Build history of the part. All positions in model axes, mm. Face numbers are marked on the shaded views. A direction names the side the tool comes from. Give positions to 0.01 mm unless a question says otherwise; leave off trailing zeros. Write each loop counter-clockwise with the first axis right and the second up, starting at its lowest first coordinate (ties: lowest second). Pieces come first, ordered by that corner, then holes. Notation, with made-up numbers: M 0.25,16.5 L 12.25,16.5 A14 cw 12.25,22.5 Z; hole C 64,41.25 d7. An arc over 180 degrees is marked long. Return JSON: item names as keys, results as strings. Group by question number.
Q1. Pull direction Y, two halves, no side cores. Call the marked faces 4, 5 and 6: +Y half, -Y half, draft (parallel to the pull), parting line (faces both ways), or undercut.
Q2. Wall check: probe 1 along Y at (x, z) = (0.25, -1.75); probe 2 along Y at (x, z) = (0, 6); probe 3 along X at (y, z) = (54, 9). Give the ranges that are in metal, low to high.
Q3. Band-saw the part on A-A, the plane x = 0. Give the cut face in (y, z), then the cut area to 3 significant figures.
Q4. Flat gauge pins, fed straight in: pin 1 Ø6 at (x, y) = (-2, -17.5) entering from -Z; pin 2 Ø6.5 at (x, y) = (0, 54) entering from +Z; pin 3 Ø10 at (x, z) = (-3.5, -5.5) entering from +Y; pin 4 Ø12 at (x, z) = (7, 11.5) entering from -Y. Where does each tip first touch, or does it go through?
Q5. Tool access for the marked faces 1, 2 and 3: list every direction of +Z, -Z, +X, -X, +Y, -Y with a clear straight run to the whole face (end or side of a thin tool).
Q6. Band-saw the part on B-B, the plane y = 5. Give the cut face in (x, z).
from build123d import *

# Parameters (mm, degrees)
CROQUIS1_R              = 4
SALIENTE_EXTRUIR1_DEPTH = 4
SALIENTE_EXTRUIR2_START = -8
CROQUIS1_5_R            = 4
SALIENTE_EXTRUIR2_DEPTH = 8
REDONDEO2_R             = 2
CROQUIS1_6_R            = 4
SALIENTE_EXTRUIR3_DEPTH = 15
REDONDEO1_START         = -10
REDONDEO1_DEPTH         = 4
REDONDEO1_START_2       = 6
REDONDEO1_2_DEPTH       = 4
REDONDEO1_START_3       = 4
REDONDEO1_3_DEPTH       = 10
REDONDEO1_START_4       = -6
REDONDEO1_4_DEPTH       = 12


with BuildPart() as part:
    # Croquis1 → Saliente-Extruir1 (new body)
    with BuildSketch(Plane.XY):
        with BuildLine():
            Line((10, 54), (10, -54))
            ThreePointArc((10, -54), (0, -64), (-10, -54))
            Line((-10, -54), (-10, 54))
            ThreePointArc((-10, 54), (0, 64), (10, 54))
        make_face()
        with Locations((0, -54)):
            Circle(CROQUIS1_R, mode=Mode.SUBTRACT)
        with BuildLine():
            Line((6, 38), (6, -38))
            ThreePointArc((6, -38), (0, -44), (-6, -38))
            Line((-6, -38), (-6, 38))
            ThreePointArc((-6, 38), (0, 44), (6, 38))
        make_face(mode=Mode.SUBTRACT)
    extrude(amount=SALIENTE_EXTRUIR1_DEPTH)

    # Croquis1<5> → Saliente-Extruir2 (add)
    with BuildSketch(Plane.XY.offset(SALIENTE_EXTRUIR2_START)):
        with BuildLine():
            Line((10, -54), (10, -47))
            Line((10, -47), (-10, -47))
            Line((-10, -47), (-10, -54))
            ThreePointArc((-10, -54), (0, -64), (10, -54))
        make_face()
        with Locations((0, -54)):
            Circle(CROQUIS1_5_R, mode=Mode.SUBTRACT)
    extrude(amount=SALIENTE_EXTRUIR2_DEPTH)

    # Redondeo2
    redondeo2_edges = [part.edges().sort_by_distance(p)[0] for p in [
        (0, -47, 0),
        (0, -47, -8),
    ]]
    fillet(redondeo2_edges, radius=REDONDEO2_R)

    # Croquis1<6> → Saliente-Extruir3 (add)
    with BuildSketch(Plane.XY):
        with BuildLine():
            Line((10, 47), (10, 54))
            ThreePointArc((10, 54), (0, 64), (-10, 54))
            Line((-10, 54), (-10, 47))
            Line((-10, 47), (10, 47))
        make_face()
        with Locations((0, 54)):
            Circle(CROQUIS1_6_R, mode=Mode.SUBTRACT)
    extrude(amount=SALIENTE_EXTRUIR3_DEPTH)

    # Redondeo1: read off the stored shape, not the designer's step
    # Redondeo1 outline → Redondeo1 (add)
    with BuildSketch(Plane.YZ.offset(REDONDEO1_START)):
        with BuildLine():
            Line((47, 4), (47, 14))
            ThreePointArc((47, 14), (44.071067812, 6.928932188), (37, 4))
            Line((37, 4), (47, 4))
        make_face()
    extrude(amount=REDONDEO1_DEPTH)

    # Redondeo1 2 outline → Redondeo1 2 (add)
    with BuildSketch(Plane.YZ.offset(REDONDEO1_START_2)):
        with BuildLine():
            Line((47, 4), (47, 14))
            ThreePointArc((47, 14), (44.071067812, 6.928932188), (37, 4))
            Line((37, 4), (47, 4))
        make_face()
    extrude(amount=REDONDEO1_2_DEPTH)

    # Redondeo1 3 outline → Redondeo1 3 (add)
    with BuildSketch(Plane.XY.offset(REDONDEO1_START_3)):
        with BuildLine():
            Line((-6, 47), (-6, 38))
            ThreePointArc((-6, 38), (0, 44), (6, 38))
            Line((6, 38), (6, 47))
            Line((6, 47), (-6, 47))
        make_face()
    extrude(amount=REDONDEO1_3_DEPTH)

    # Redondeo1 4 outline → Redondeo1 4 (cut)
    with BuildSketch(Plane.YZ.offset(REDONDEO1_START_4)):
        with BuildLine():
            ThreePointArc((37, 4), (44.071067812, 6.928932188), (47, 14))
            Line((47, 14), (37, 14))
            Line((37, 14), (37, 4))
        make_face()
    extrude(amount=REDONDEO1_4_DEPTH, mode=Mode.SUBTRACT)


solid = part.part
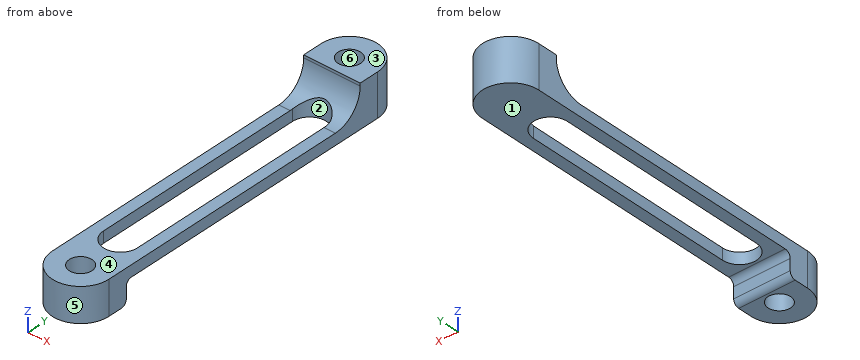
From the geometry:
{
 "1": {"face 4": "draft", "face 5": "-Y half", "face 6": "undercut"},
 "2": {"probe 1": "y = -64 to -57.99, -50.01 to -46.98", "probe 2": "y = 44 to 50, 58 to 64", "probe 3": "x = -10 to -4, 4 to 10"},
 "3": {"outline": "M -64,-8 L -58,-8 L -58,4 L -64,4 Z; M -50,-8 L -49,-8 A2 ccw -47,-6 L -47,-2 A2 cw -45,0 L -44,0 L -44,4 L -50,4 Z; M 44,0 L 64,0 L 64,15 L 58,15 L 58,4 L 50,4 L 50,15 L 47,15 L 47,14 A10 cw 44,6.86 Z", "area": "314 mm^2"},
 "4": {"pin 1": "passes through", "pin 2": "stops at z = 4", "pin 3": "stops at y = -46.32", "pin 4": "stops at y = 42.27"},
 "5": {"face 1": "-Z, +X, -X, +Y", "face 2": "+Z, -Z", "face 3": "+Z, +X, -X, +Y, -Y"},
 "6": {"outline": "M -10,0 L -6,0 L -6,4 L -10,4 Z; M 6,0 L 10,0 L 10,4 L 6,4 Z"}
}
